CAD build for the part. Positions are in the model's coordinates, mm. Face numbers are marked on the shaded views. A direction names the side the tool comes from. Coordinates: 2 decimals unless noted, no trailing zeros. Return JSON: item names as keys, results as strings.
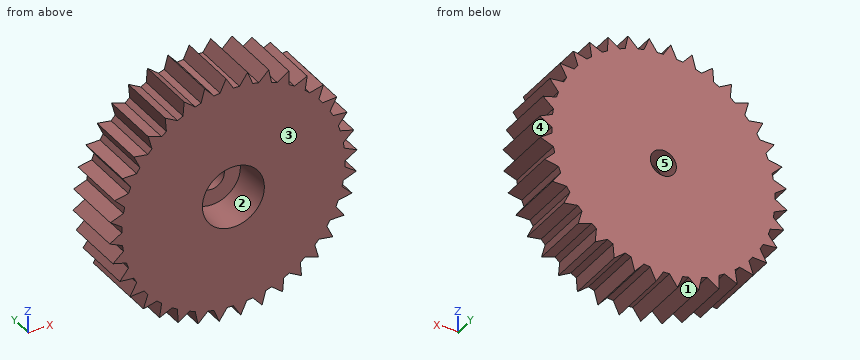
from build123d import *

# Parameters (mm, degrees)
SKETCH1_R           = 9
BOSS_EXTRUDE1_DEPTH = 5
SKETCH2_R           = 2.5
CUT_EXTRUDE1_DEPTH  = 3
CUT_EXTRUDE1_DRAFT  = -3
SKETCH3_R           = 1.05
CUT_EXTRUDE2_DEPTH  = 3
BOSS_EXTRUDE2_DEPTH = 5


with BuildPart() as part:
    # Sketch1 → Boss-Extrude1 (new body)
    with BuildSketch(Plane(origin=(0, 0, 0), x_dir=(1, 0, 0), z_dir=(0, 1, 0))):
        with Locations(Location((0, 0, 0), (0, 0, 270))):
            Circle(SKETCH1_R)
    extrude(amount=BOSS_EXTRUDE1_DEPTH)


with BuildPart() as cut_extrude1_tool:
    # Sketch2 → Cut-Extrude1 (with draft: the straight prism first)
    with BuildSketch(Plane.XZ):
        Circle(SKETCH2_R)
    extrude(amount=-CUT_EXTRUDE1_DEPTH)
    # Cut-Extrude1: the draft: its side faces are tilted about the plane it starts from
    cut_extrude1_sides = [cut_extrude1_tool.faces().sort_by_distance(p)[0] for p in [
        (-2.5, 1.5, 0),
    ]]
    draft(cut_extrude1_sides, Plane.XZ, CUT_EXTRUDE1_DRAFT)


with BuildPart() as part_1:
    add(part.part)

    # Cut-Extrude1: cut by cut_extrude1_tool
    add(cut_extrude1_tool.part, mode=Mode.SUBTRACT)

    # Sketch3 → Cut-Extrude2 (cut)
    with BuildSketch(Plane.XZ.offset(-3)):
        with Locations(Location((0, 0, 0), (0, 0, 270))):
            Circle(SKETCH3_R)
    extrude(amount=-CUT_EXTRUDE2_DEPTH, mode=Mode.SUBTRACT)

    # Sketch4 → Boss-Extrude2 (add)
    with BuildSketch(Plane(origin=(0, 5, 0), x_dir=(1, 0, 0), z_dir=(0, 1, 0))):
        Polygon((0, 9), (0.59385284, 9.966251069), (1.073329801, 8.935768749), align=None)
        Polygon((1.562833599, 8.863269777), (2.315452217, 9.711719857), (2.608703469, 8.613632579), align=None)
        Polygon((3.07818129, 8.457233587), (3.966697751, 9.162102953), (4.064813002, 8.029775542), align=None)
        Polygon((4.5, 7.794228634), (5.49741718, 8.334100186), (5.397415249, 7.201937839), align=None)
        Polygon((5.785088487, 6.894399988), (6.86110037, 7.252870002), (6.566019765, 6.155272898), align=None)
        Polygon((6.894399988, 5.785088487), (8.016312498, 5.951265034), (7.535119092, 4.921583105), align=None)
        Polygon((7.794228634, 4.5), (8.927953026, 4.468833889), (8.27526764, 3.5383535), align=None)
        Polygon((8.457233587, 3.07818129), (9.56832222, 2.850619487), (8.763976367, 2.047612815), align=None)
        Polygon((8.863269777, 1.562833599), (9.917962784, 1.145790455), (8.986396107, 0.49465645), align=None)
        Polygon((9, 0), (9.966251069, -0.59385284), (8.935768749, -1.073329801), align=None)
        Polygon((8.863269777, -1.562833599), (9.711719857, -2.315452217), (8.613632579, -2.608703469), align=None)
        Polygon((8.457233587, -3.07818129), (9.162102953, -3.966697751), (8.029775542, -4.064813002), align=None)
        Polygon((7.794228634, -4.5), (8.334100186, -5.49741718), (7.201937839, -5.397415249), align=None)
        Polygon((6.894399988, -5.785088487), (7.252870002, -6.86110037), (6.155272898, -6.566019765), align=None)
        Polygon((5.785088487, -6.894399988), (5.951265034, -8.016312498), (4.921583105, -7.535119092), align=None)
        Polygon((4.5, -7.794228634), (4.468833889, -8.927953026), (3.5383535, -8.27526764), align=None)
        Polygon((3.07818129, -8.457233587), (2.850619487, -9.56832222), (2.047612815, -8.763976367), align=None)
        Polygon((1.562833599, -8.863269777), (1.145790455, -9.917962784), (0.49465645, -8.986396107), align=None)
        Polygon((0, -9), (-0.59385284, -9.966251069), (-1.073329801, -8.935768749), align=None)
        Polygon((-1.562833599, -8.863269777), (-2.315452217, -9.711719857), (-2.608703469, -8.613632579), align=None)
        Polygon((-3.07818129, -8.457233587), (-3.966697751, -9.162102953), (-4.064813002, -8.029775542), align=None)
        Polygon((-4.5, -7.794228634), (-5.49741718, -8.334100186), (-5.397415249, -7.201937839), align=None)
        Polygon((-5.785088487, -6.894399988), (-6.86110037, -7.252870002), (-6.566019765, -6.155272898), align=None)
        Polygon((-6.894399988, -5.785088487), (-8.016312498, -5.951265034), (-7.535119092, -4.921583105), align=None)
        Polygon((-7.794228634, -4.5), (-8.927953026, -4.468833889), (-8.27526764, -3.5383535), align=None)
        Polygon((-8.457233587, -3.07818129), (-9.56832222, -2.850619487), (-8.763976367, -2.047612815), align=None)
        Polygon((-8.863269777, -1.562833599), (-9.917962784, -1.145790455), (-8.986396107, -0.49465645), align=None)
        Polygon((-9, 0), (-9.966251069, 0.59385284), (-8.935768749, 1.073329801), align=None)
        Polygon((-8.863269777, 1.562833599), (-9.711719857, 2.315452217), (-8.613632579, 2.608703469), align=None)
        Polygon((-8.457233587, 3.07818129), (-9.162102953, 3.966697751), (-8.029775542, 4.064813002), align=None)
        Polygon((-7.794228634, 4.5), (-8.334100186, 5.49741718), (-7.201937839, 5.397415249), align=None)
        Polygon((-6.894399988, 5.785088487), (-7.252870002, 6.86110037), (-6.155272898, 6.566019765), align=None)
        Polygon((-5.785088487, 6.894399988), (-5.951265034, 8.016312498), (-4.921583105, 7.535119092), align=None)
        Polygon((-4.5, 7.794228634), (-4.468833889, 8.927953026), (-3.5383535, 8.27526764), align=None)
        Polygon((-3.07818129, 8.457233587), (-2.850619487, 9.56832222), (-2.047612815, 8.763976367), align=None)
        Polygon((-1.562833599, 8.863269777), (-1.145790455, 9.917962784), (-0.49465645, 8.986396107), align=None)
    extrude(amount=-BOSS_EXTRUDE2_DEPTH)


solid = part_1.part
Item 1: Which spindle directions (+Z, -Z, +X, -X, +Y, -Y) get a long thin tool onto all of the face, cutting with end or side? Do the marked faces 4 and 5. Say none if no direction does.
Findings below:
{"face 4": "+X, +Y, -Y", "face 5": "+Y, -Y"}
Item 2: Drop flat-ended pins along their axis: P1, Ø3, axis at y = 3.5, z = 7, coming from the -X side; P2, Ø3, axis at y = 2, z = -0.5, coming from the +X side. Give the stop position or say it passes through.
Findings below:
{"P1": "stops at x = -8.02", "P2": "stops at x = 9.97"}
Item 3: Mould opens along Z. For the marked faces 1, 2 and 3 say: released by +Z, released by -Z, zero draft, split by the parting line, or undercut.
Findings below:
{"face 1": "released by -Z", "face 2": "undercut", "face 3": "zero draft"}
Item 4: Wall check: L1, parallel to Z at x = -1, y = 0.5; L2, parallel to Z at x = 6.25, y = 2.7; L3, parallel to Z at x = 2, y = 4.5. Give the ranges that are in metal, low to high. Write a range as [from, to].
Findings below:
{"L1": "z = [-9.71, -2.26], [2.26, 9.09]", "L2": "z = [-7.05, 6.59]", "L3": "z = [-9.36, 8.77]"}
